from build123d import *

# Parameters (mm, degrees)
F2_DEPTH = 5


with BuildPart() as f2:
    # F1 (on Right) → F2 (new body)
    with BuildSketch(Plane.YZ):
        Polygon((0, 15), (0, 0), (30, 0), (30, -5), (35, -5), (35, 0), (43.5, 0), (43.5, 2), (42.25, 2), (42.25, 5), (43.5, 5), (43.5, 6), (46.5, 6), (46.5, 5), (47.75, 5), (47.75, 2), (46.5, 2), (46.5, 0), (55, 0), (55, -5), (60, -5), (60, 0), (90, 0), (90, 15), (95, 15), (95, 20), (90, 20), (90, 28.5), (88, 28.5), (88, 27.25), (85, 27.25), (85, 28.5), (84, 28.5), (84, 31.5), (85, 31.5), (85, 32.75), (88, 32.75), (88, 31.5), (90, 31.5), (90, 40), (95, 40), (95, 45), (90, 45), (90, 60), (60, 60), (60, 65), (55, 65), (55, 60), (46.5, 60), (46.5, 58), (47.75, 58), (47.75, 55), (46.5, 55), (46.5, 54), (43.5, 54), (43.5, 55), (42.25, 55), (42.25, 58), (43.5, 58), (43.5, 60), (35, 60), (35, 65), (30, 65), (30, 60), (0, 60), (0, 45), (-5, 45), (-5, 40), (0, 40), (0, 31.5), (2, 31.5), (2, 32.75), (5, 32.75), (5, 31.5), (6, 31.5), (6, 28.5), (5, 28.5), (5, 27.25), (2, 27.25), (2, 28.5), (0, 28.5), (0, 20), (-5, 20), (-5, 15), align=None)
    extrude(amount=F2_DEPTH)


solid = f2.part
For this review, take the finished solid that the model builds, in its own axes (mm). A direction names the side the tool comes from. Give positions to 0.01 mm unless a question says otherwise; leave off trailing zeros. Order: outer loops, then holes, each group sorted by start corner. A loop starts at its lowest first (then second) coordinate and runs counter-clockwise, first axis right, second up. Notation, with made-up numbers: (76, 88.5) -> (103, 88.5) arc R22 cw to (103, 95.5) -> close; hole circle Ø8 at (-34, 8). An arc over 180 degrees is marked (long way). Write item = value, one per line.
1) We need section A-A, the plane y = 78. Give the boundary of the cut face in (x, z).
Findings:
outline = (0, 0) -> (5, 0) -> (5, 60) -> (0, 60) -> close
2) We need section B-B, the plane z = 52. Give the boundary of the cut face in (x, y).
Findings:
outline = (0, 0) -> (5, 0) -> (5, 90) -> (0, 90) -> close
3) Draft analysis for pull direction Z (two halves, no side actions). For faces 5 (the face through (2, 93, 45)), 6 (the face through (2, 95, 17)), 7 (the face through (2, 93, 20)), 8 (the face through (2, 57, -5)), state which applies: pulls with the +Z half, pulls with the -Z half, needs draft (parallel to the pull), parting line crosses it, or undercut.
Findings:
face_5 = pulls with the +Z half
face_6 = needs draft
face_7 = undercut
face_8 = pulls with the -Z half
4) Insertion check: pin 1 (0.6 mm diameter, centred on x = 1.5, y = 1, fed in from -Z); pin 2 (2.5 mm diameter, centred on x = 1.5, z = 36, fed in from +Y); pin 3 (2.5 mm diameter, centred on x = 2, z = -3, fed in from -Y). Each pin has a flat end and moves straight along its axis. Give the tip position at first contact, or say it passes through.
Findings:
pin_1 = 0
pin_2 = 90
pin_3 = 30
5) To check wall thickness, follow L1, parallel to Y at x = 3.95, z = 28; L2, parallel to Z at x = 2.75, y = 85.5; L3, parallel to Y at x = 3.45, z = 5.5. State the ranges of each line that lie inside material, in increasing order. Write a range as from..to.
Findings:
L1 = 0..2, 5..85, 88..90
L2 = 0..27.25, 32.75..60
L3 = 0..43.5, 46.5..90
6) For faces 1 (the face through (2, 60, -3)), 2 (the face through (2, 86, 32.75)), 3 (the face through (2, 46.5, 59)), 4 (the face through (2, -3, 15)), list the 3-axis set-ups (+Z, -Z, +X, -X, +Y, -Y) from which the entire face can be reached by the end or side of a thin tool; tool diameter is ignored.
Findings:
face_1 = -Z, +X, -X, +Y
face_2 = +X, -X
face_3 = +Z, +X, -X
face_4 = -Z, +X, -X, -Y
